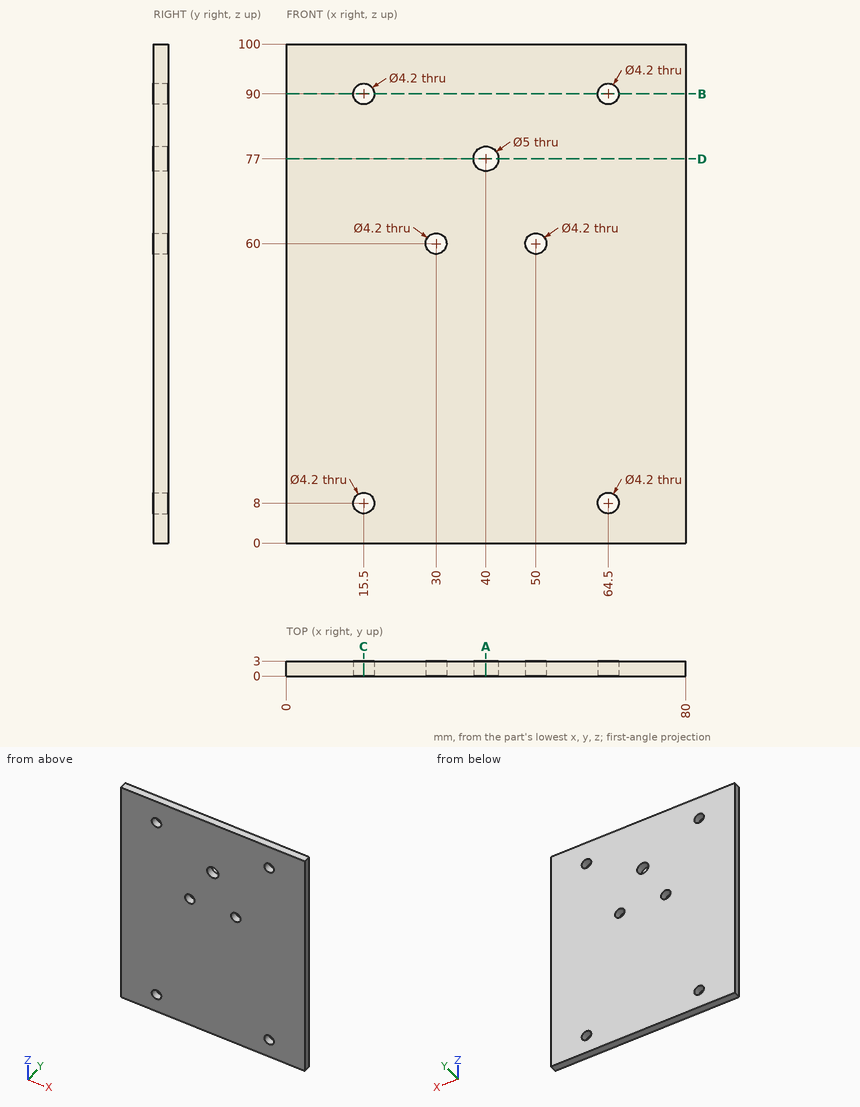
Print and shaded views of the part. All mm, measured from the part's lowest x, y and z. Round coordinates to 2 decimals unless told otherwise and drop trailing zeros. Write each loop counter-clockwise with the first axis right and the second up, starting at its lowest first coordinate (ties: lowest second). Pieces come first, ordered by that corner, then holes. Notation, with made-up numbers: M 30.25,76 L 42.25,76 A14 cw 42.25,102 Z; hole C 10,10 d6. An arc over 180 degrees is marked long. Use a Markdown table: item, result. Add a question column.
1. Drill centre lines: probe 1 along X at (y, z) = (1.6, 8); probe 2 along X at (y, z) = (0.85, 60); probe 3 along Z at (x, y) = (38.5, 2.25). Where is each one in solid material? Low to high.
2. Slice it at A-A on x = 40. Give the cut face in (y, z).
3. Slice it at C-C on x = 15.5. Give the cut face in (y, z).
4. Flat gauge pin, fed straight in: P1, Ø3.5, axis at x = 30, z = 60, coming from the -Y side (3 decimals). Where does the tip first touch, or does it go through?
5. Slice it at B-B on z = 90. Give the cut face in (x, y), then the cut area to 3 significant figures.
6. Slice it at D-D on z = 77. Give the cut face in (x, y), then the cut area to 3 significant figures.
Reply:
| question | item | result |
|---|---|---|
| 1 | probe 1 | x = 0 to 13.4, 17.6 to 62.4, 66.6 to 80 |
| 1 | probe 2 | x = 0 to 27.9, 32.1 to 47.9, 52.1 to 80 |
| 1 | probe 3 | z = 0 to 75, 79 to 100 |
| 2 | outline | M 0,0 L 3,0 L 3,74.5 L 0,74.5 Z; M 0,79.5 L 3,79.5 L 3,100 L 0,100 Z |
| 3 | outline | M 0,0 L 3,0 L 3,5.9 L 0,5.9 Z; M 0,10.1 L 3,10.1 L 3,87.9 L 0,87.9 Z; M 0,92.1 L 3,92.1 L 3,100 L 0,100 Z |
| 4 | P1 | passes through |
| 5 | outline | M 0,0 L 13.4,0 L 13.4,3 L 0,3 Z; M 17.6,0 L 62.4,0 L 62.4,3 L 17.6,3 Z; M 66.6,0 L 80,0 L 80,3 L 66.6,3 Z |
| 5 | area | 215 mm^2 |
| 6 | outline | M 0,0 L 37.5,0 L 37.5,3 L 0,3 Z; M 42.5,0 L 80,0 L 80,3 L 42.5,3 Z |
| 6 | area | 225 mm^2 |
